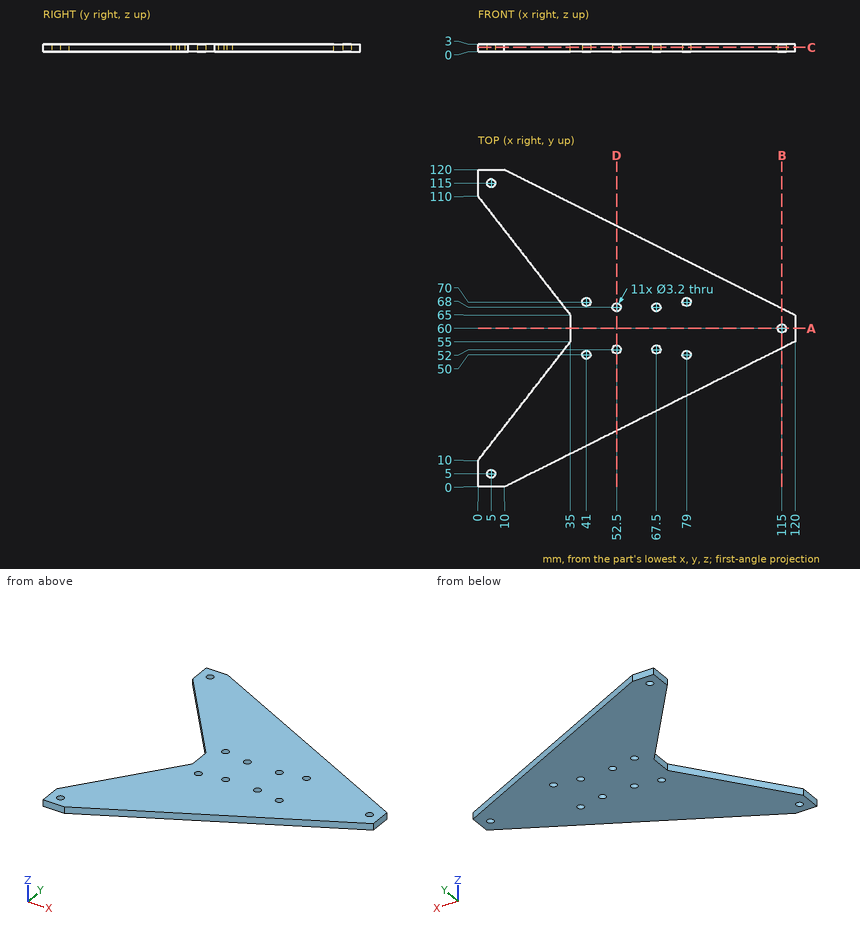
Source: three-view drawing plus pictorial views. Frame: mm from the lowest corner of the part. Coordinates: 2 decimals unless noted, no trailing zeros. Write each loop counter-clockwise with the first axis right and the second up, starting at its lowest first coordinate (ties: lowest second). Pieces come first, ordered by that corner, then holes. Notation, with made-up numbers: (21, -30.75) - (42, -30.75) arc R13 ccw to (42, -26.75) - close; hole circle Ø4 at (-4.75, 82). An arc over 180 degrees is marked (long way). Return JSON: item names as keys, results as strings.
Item 1: Section query A-A (y = 60). Output: boundary loops of the cut face in (x, z).
Completed:
{"outline": "(35, 0) - (113.4, 0) - (113.4, 3) - (35, 3) - close; (116.6, 0) - (120, 0) - (120, 3) - (116.6, 3) - close"}
Item 2: Section query B-B (x = 115). Output: boundary loops of the cut face in (y, z), and give its area (3 significant figures).
Completed:
{"outline": "(52.5, 0) - (58.4, 0) - (58.4, 3) - (52.5, 3) - close; (61.6, 0) - (67.5, 0) - (67.5, 3) - (61.6, 3) - close", "area": "35.4 mm2"}
Item 3: Section query D-D (x = 52.5). Output: boundary loops of the cut face in (y, z), and give its area (3 significant figures).
Completed:
{"outline": "(21.25, 0) - (50.4, 0) - (50.4, 3) - (21.25, 3) - close; (53.6, 0) - (66.4, 0) - (66.4, 3) - (53.6, 3) - close; (69.6, 0) - (98.75, 0) - (98.75, 3) - (69.6, 3) - close", "area": "213 mm2"}
Item 4: Pin query (flat end, axial travel): pin 1 Ø1 at (y, z) = (103, 1) entering from -X; pin 2 Ø1.5 at (y, z) = (58, 1.5) entering from -X; pin 3 Ø1 at (y, z) = (67, 2) entering from -X. Return the tip coordinate at first contact, or that it passes through.
Completed:
{"pin 1": "stops at x = 5.06", "pin 2": "stops at x = 35", "pin 3": "stops at x = 33.06"}
Item 5: Section query C-C (z = 1.75). Count the separate pieces of the cut face and the enclosed holes in it, and give its area (3 significant figures).
Completed:
{"separate pieces": "1", "enclosed holes": "11", "area": "6,340 mm2"}
Item 6: Line query: L1, parallel to Y at x = 67.5, z = 2.4; L2, parallel to X at y = 52, z = 1.85; L3, parallel to Y at x = 79, z = 1.25. Output: solid intervals per line, ascending.
Completed:
{"L1": "y = 28.75 to 50.4, 53.6 to 66.4, 69.6 to 91.25", "L2": "x = 32.67 to 50.9, 54.1 to 65.9, 69.1 to 114", "L3": "y = 34.5 to 48.4, 51.6 to 68.4, 71.6 to 85.5"}
